The listing builds one solid part. Answer for the finished solid, in the listing's coordinates (mm). A direction names the side the tool comes from. Give positions to 0.01 mm unless a question says otherwise; leave off trailing zeros. Order: outer loops, then holes, each group sorted by start corner. A loop starts at its lowest first (then second) coordinate and runs counter-clockwise, first axis right, second up. Notation, with made-up numbers: (44, -14) - (73, -14) arc R21 ccw to (73, -4) - close; hole circle Ø5 at (-24.75, 39). An arc over 180 degrees is marked (long way). Answer as CSV lines item,"result". Start each with the question number.
1. Flat-ended cylindrical pins translate along their axes: pin 1 (4.5 mm diameter, centred on x = -18.38, z = 18.38, fed in from +Y); pin 2 (10.5 mm diameter, centred on x = -25.11, z = 6.73, fed in from -Y); pin 3 (3 mm diameter, centred on x = 3, z = -32.5, fed in from +Y); pin 4 (3 mm diameter, centred on x = 18.38, z = 18.38, fed in from +Y). Find the tip coordinate at first contact, or state that the pin passes through.
2. Determine the mould class of faces 1 (the cylindrical face through (31.09, 2.47, 18.15)), 2 (the cylindrical face through (11.866, 7.958, 5.587)), 3 (the cylindrical face through (28.214, 3.521, 5.753)) for opening direction Z: +Z half, -Z half, draft (parallel to the pull), parting line (faces both ways), or undercut.
3. Consider line 1 along Z through (x, y) = (3, 0.75); line 2 along X through (y, z) = (2.25, -9); line 3 along X through (y, z) = (4, 18). Determine where each line is inside the solid, lowest interval first. Write a range as [from, to].
4. Section B-B on z = -8.5 is taken. Give the vertices of the cut face in (x, y), and give its area (3 significant figures).
5. Section A-A on z = 0 is taken. Give the vertices of the cut face in (x, y).
6. Which of the six approach directions +Z, -Z, +X, -X, +Y, -Y give full straight-line access (tool end or side, diameter ignored) to faces 4 (the cylindrical face through (6.025, 3.521, -21.941)), 5 (the cylindrical face through (23.86, 1.01, 5.58))?
7. Section D-D on y = 4 is taken. Count the separate pieces of the cut face and the enclosed holes in it, and give its area (3 significant figures).
8. Section C-C on z = -18 is taken. Give the vertices of the cut face in (x, y), and give its area (3 significant figures).
from build123d import *

# Parameters (mm, degrees)
SKETCH1_R           = 36
SKETCH1_R_2         = 13
BOSS_EXTRUDE1_DEPTH = 5
SKETCH2_R           = 1.65
CUT_EXTRUDE1_DEPTH  = 6
CIRPATTERN1_COUNT   = 3
SKETCH3_R           = 76.029468034
CUT_EXTRUDE2_DEPTH  = 10
CIRPATTERN2_COUNT   = 3
FILLET1_R           = 1
SKETCH4_R           = 5.05
BOSS_EXTRUDE2_DEPTH = 6
SKETCH7_R           = 3.25
CUT_EXTRUDE5_DEPTH  = 3.2
CIRPATTERN3_COUNT   = 3
SKETCH8_R           = 1.5
CUT_EXTRUDE6_DEPTH  = 10
SKETCH12_R          = 2
CUT_EXTRUDE8_DEPTH  = 12.0000001
CIRPATTERN4_COUNT   = 3
SKETCH13_R          = 1.7
CUT_EXTRUDE9_DEPTH  = 6.0000001
CIRPATTERN5_COUNT   = 3
SKETCH14_R          = 3.25
CUT_EXTRUDE10_DEPTH = 3


with BuildPart() as part:
    # Sketch1 → Boss-Extrude1 (new body)
    with BuildSketch(Plane(origin=(0, 0, 0), x_dir=(1, 0, 0), z_dir=(0, 1, 0))):
        Circle(SKETCH1_R)
        Circle(SKETCH1_R_2, mode=Mode.SUBTRACT)
    extrude(amount=BOSS_EXTRUDE1_DEPTH)

    # Sketch2 → Cut-Extrude1 (cut, through all)
    with BuildSketch(Plane(origin=(0, 5, 0), x_dir=(1, 0, 0), z_dir=(0, 1, 0))):
        with Locations((2.788983768, 31.878230339)):
            Circle(SKETCH2_R)
    cut_extrude1 = extrude(amount=-CUT_EXTRUDE1_DEPTH, mode=Mode.SUBTRACT)

    # CirPattern1: Cut-Extrude1 ×3 about axis
    cirpattern1_axis = Axis((0, 0, 0), (0, 1, 0))
    for i in range(1, CIRPATTERN1_COUNT):
        add(cut_extrude1.rotate(cirpattern1_axis, i * 360 / CIRPATTERN1_COUNT), mode=Mode.SUBTRACT)

    # Sketch3 → Cut-Extrude2 (cut)
    with BuildSketch(Plane(origin=(0, 5, 0), x_dir=(1, 0, 0), z_dir=(0, 1, 0))):
        with Locations((86.602540378, 50)):
            Circle(SKETCH3_R)
    cut_extrude2 = extrude(amount=-CUT_EXTRUDE2_DEPTH, mode=Mode.SUBTRACT)

    # CirPattern2: Cut-Extrude2 ×3 about axis
    cirpattern2_axis = Axis((0, 0, 0), (0, 1, 0))
    for i in range(1, CIRPATTERN2_COUNT):
        add(cut_extrude2.rotate(cirpattern2_axis, i * 360 / CIRPATTERN2_COUNT), mode=Mode.SUBTRACT)

    # Fillet1
    fillet1_edges = [part.edges().sort_by_distance(p)[0] for p in [
        (12.31272516, 2.5, -33.828934348),
        (35.453079108, 2.5, 6.251334396),
        (23.140353949, 2.5, 27.577599952),
        (-23.140353949, 2.5, 27.577599952),
        (-35.453079108, 2.5, 6.251334396),
        (-12.31272516, 2.5, -33.828934348),
    ]]
    fillet(fillet1_edges, radius=FILLET1_R)

    # Sketch4 → Boss-Extrude2 (add)
    with BuildSketch(Plane(origin=(0, 5, 0), x_dir=(1, 0, 0), z_dir=(0, 1, 0))):
        with Locations((0, 18)):
            Circle(SKETCH4_R)
    boss_extrude2 = extrude(amount=BOSS_EXTRUDE2_DEPTH)

    # Sketch7 → Cut-Extrude5 (cut)
    with BuildSketch(Plane(origin=(0, 5, 0), x_dir=(1, 0, 0), z_dir=(0, 1, 0))):
        with Locations((2.788983768, 31.878230339)):
            Circle(SKETCH7_R)
    cut_extrude5 = extrude(amount=-CUT_EXTRUDE5_DEPTH, mode=Mode.SUBTRACT)

    # CirPattern3: Boss-Extrude2, Cut-Extrude5 ×3 about axis
    cirpattern3_axis = Axis((0, 0, 0), (0, 1, 0))
    for i in range(1, CIRPATTERN3_COUNT):
        add(boss_extrude2.rotate(cirpattern3_axis, i * 360 / CIRPATTERN3_COUNT))
        add(cut_extrude5.rotate(cirpattern3_axis, i * 360 / CIRPATTERN3_COUNT), mode=Mode.SUBTRACT)

    # Sketch8 → Cut-Extrude6 (cut)
    with BuildSketch(Plane(origin=(0, 5, 0), x_dir=(1, 0, 0), z_dir=(0, 1, 0))):
        with Locations((14.722431864, 8.5)):
            Circle(SKETCH8_R)
    cut_extrude6 = extrude(amount=-CUT_EXTRUDE6_DEPTH, mode=Mode.SUBTRACT)

    # Sketch12 → Cut-Extrude8 (cut, through all)
    with BuildSketch(Plane(origin=(0, 11, 0), x_dir=(1, 0, 0), z_dir=(0, 1, 0))):
        with Locations((0, 18)):
            Circle(SKETCH12_R)
    cut_extrude8 = extrude(amount=-CUT_EXTRUDE8_DEPTH, mode=Mode.SUBTRACT)

    # CirPattern4: Cut-Extrude6, Cut-Extrude8 ×3 about axis
    cirpattern4_axis = Axis((0, 0, 0), (0, 1, 0))
    for i in range(1, CIRPATTERN4_COUNT):
        add(cut_extrude6.rotate(cirpattern4_axis, i * 360 / CIRPATTERN4_COUNT), mode=Mode.SUBTRACT)
        add(cut_extrude8.rotate(cirpattern4_axis, i * 360 / CIRPATTERN4_COUNT), mode=Mode.SUBTRACT)

    # Sketch13 → Cut-Extrude9 (cut, through all)
    with BuildSketch(Plane(origin=(0, 5, 0), x_dir=(1, 0, 0), z_dir=(0, 1, 0))):
        with Locations((6.729295173, 25.114071484)):
            Circle(SKETCH13_R)
        with Locations((-6.729295173, 25.114071484)):
            Circle(SKETCH13_R)
    cut_extrude9 = extrude(amount=-CUT_EXTRUDE9_DEPTH, mode=Mode.SUBTRACT)

    # CirPattern5: Cut-Extrude9 ×3 about axis
    cirpattern5_axis = Axis((0, 0, 0), (0, 1, 0))
    for i in range(1, CIRPATTERN5_COUNT):
        add(cut_extrude9.rotate(cirpattern5_axis, i * 360 / CIRPATTERN5_COUNT), mode=Mode.SUBTRACT)

    # Sketch14 → Cut-Extrude10 (cut)
    with BuildSketch(Plane(origin=(0, 5, 0), x_dir=(1, 0, 0), z_dir=(0, 1, 0))):
        with Locations((-18.384776311, -18.384776311)):
            Circle(SKETCH14_R)
        with Locations((-25.114071484, -6.729295173)):
            Circle(SKETCH14_R)
        with Locations((-6.729295173, 25.114071484)):
            Circle(SKETCH14_R)
        with Locations((6.729295173, 25.114071484)):
            Circle(SKETCH14_R)
        with Locations((25.114071484, -6.729295173)):
            Circle(SKETCH14_R)
        with Locations((18.384776311, -18.384776311)):
            Circle(SKETCH14_R)
    extrude(amount=-CUT_EXTRUDE10_DEPTH, mode=Mode.SUBTRACT)


solid = part.part
Checks:
1,pin 1,"stops at y = 2"
1,pin 2,"stops at y = 0"
1,pin 3,"stops at y = 1.8"
1,pin 4,"passes through"
2,face 1,"+Z half"
2,face 2,"parting line"
2,face 3,"undercut"
3,line 1,"z = [-35.87, -33.51], [-30.24, -12.65], [12.65, 24.03]"
3,line 2,"x = [-22.58, -16.14], [-13.31, -9.38], [9.38, 13.31], [16.14, 22.58]"
3,line 3,"x = [-31.18, -21.61], [-15.16, -1.12], [1.12, 15.16], [21.61, 22.98], [29.44, 31.18]"
4,outline,"(-22.9, 0) - (-16.22, 0) - (-16.22, 5) - (-22.9, 5) - close; (-13.22, 0) - (-9.84, 0) - (-9.84, 5) - (-13.22, 5) - close; (9.84, 0) - (13.22, 0) - (13.22, 5) - (9.84, 5) - close; (16.22, 0) - (22.9, 0) - (22.9, 5) - (16.22, 5) - close"
4,area,"101 mm²"
5,outline,"(-29.33, 0) - (-13, 0) - (-13, 5) - (-29.33, 5) - close; (13, 0) - (29.33, 0) - (29.33, 5) - (13, 5) - close"
6,face 4,"+Y"
6,face 5,"+Y, -Y"
7,separate pieces,"1"
7,enclosed holes,"16"
7,area,"2,050 mm²"
8,outline,"(-17.64, 0) - (-2, 0) - (-2, 11) - (-5.05, 11) - (-5.05, 5) - (-17.64, 5) - close; (2, 0) - (17.64, 0) - (17.64, 5) - (5.05, 5) - (5.05, 11) - (2, 11) - close"
8,area,"193 mm²"
